from build123d import *

# Parameters (mm, degrees)
SKETCH1_W                = 22.575
SKETCH1_H                = 18
SKETCH1_R                = 2.75
BOSS_EXTRUDE1_DEPTH      = 4
BOSS_EXTRUDE1_DEPTH_BACK = 4
SKETCH3_R                = 3.375
SKETCH3_R_2              = 0.9905
CUT_EXTRUDE1_DEPTH       = 19
SKETCH4_W                = 13.55
SKETCH4_H                = 3.5
CUT_EXTRUDE2_DEPTH       = 19
CUT_EXTRUDE3_DEPTH       = 5.5
CHAMFER1_SIZE            = 2


with BuildPart() as part:
    # Sketch1 → Boss-Extrude1 (new body, two sides)
    with BuildSketch(Plane(origin=(0, 0, 0), x_dir=(1, 0, 0), z_dir=(0, 1, 0))) as boss_extrude1_sk:
        with Locations((-4.0875, 0)):
            Rectangle(SKETCH1_W, SKETCH1_H)
        Circle(SKETCH1_R, mode=Mode.SUBTRACT)
    extrude(amount=BOSS_EXTRUDE1_DEPTH)
    extrude(boss_extrude1_sk.sketch, amount=-BOSS_EXTRUDE1_DEPTH_BACK)

    # Sketch3 → Cut-Extrude1 (cut, through all)
    with BuildSketch(Plane.XY.offset(9)):
        with Locations((-11, 0)):
            Circle(SKETCH3_R)
        with Locations((-6.417424305, -2)):
            Circle(SKETCH3_R_2)
    extrude(amount=-CUT_EXTRUDE1_DEPTH, mode=Mode.SUBTRACT)

    # Sketch4 → Cut-Extrude2 (cut, through all)
    with BuildSketch(Plane.XY.offset(9)):
        with Locations((0.425, 2.25)):
            Rectangle(SKETCH4_W, SKETCH4_H)
    extrude(amount=-CUT_EXTRUDE2_DEPTH, mode=Mode.SUBTRACT)

    # Sketch5 → Cut-Extrude3 (cut, through all)
    with BuildSketch(Plane(origin=(0, 0.5, 0), x_dir=(-1, 0, 0), z_dir=(0, 1, 0))):
        Polygon((-1.2, -9), (-7.2, -3), (-7.2, -9), align=None)
        Polygon((-1.2, 9), (-7.2, 3), (-7.2, 9), align=None)
    extrude(amount=-CUT_EXTRUDE3_DEPTH, mode=Mode.SUBTRACT)

    # Chamfer1
    chamfer1_edges = [part.edges().sort_by_distance(p)[0] for p in [
        (-15.375, 4, 0),
        (-15.375, -4, 0),
        (-6.35, 4, 0),
    ]]
    chamfer(chamfer1_edges, length=CHAMFER1_SIZE)


solid = part.part
Can you work these out from the model? Positions are in its coordinate system, mm. A direction names the side the tool comes from. Round coordinates to 2 decimals unless told otherwise and drop trailing zeros. Write each loop counter-clockwise with the first axis right and the second up, starting at its lowest first coordinate (ties: lowest second). Pieces come first, ordered by that corner, then holes. Notation, with made-up numbers: (45.5, 65.5) - (91.5, 65.5) arc R17 ccw to (91.5, 71.5) - close; hole circle Ø5 at (78, -8). An arc over 180 degrees is marked (long way). Write each question's results on one line, items separated by ' | '. Start each with the question number.
1) Suppose I cut it at B-B (x = 0). List the corners of the cut face in (y, z) for me, and give its area (4 significant figures).
2) For pin 1 Ø2 at (x, z) = (-4.5, 2.5) entering from +Y; pin 2 Ø2.5 at (x, y) = (-6.42, -2) entering from +Z; pin 3 Ø0.8 at (y, z) = (1.5, -2.5) entering from +X; pin 4 Ø4.5 at (x, z) = (0, 0) entering from +Y, each with a flat end and sliding along its axis, tell me the tip position at first contact or that it passes through.
3) We'd pull the mould along X, two halves only. Please class faces 3 (the flat face through (-7.34, 2.99, 0.13)), 4 (the cylindrical face through (-7.407, -1.956, 0.126)), 5 (the flat face through (-14.361, -3.014, 0.126)): released by +X, released by -X, zero draft, split by the parting line, or undercut.
4) Suppose I cut it at C-C (y = -2.5). List the corners of the cut face in (x, z) for me (3 decimals).
5) Suppose I cut it at A-A (z = 0). Give the number of separate pieces and of enclosed holes in the cut face, and give its area (3 significant figures).
6) Please list where these lines run through material, in increasing order: line 1 (X direction, y = -2.5, z = 6) (3 decimals); line 2 (X direction, y = -1.6, z = 0) (3 decimals); line 3 (X direction, y = -2.75, z = -1.25) (3 decimals).
7) Which directions (+Z, -Z, +X, -X, +Y, -Y) give clear straight access to the entire face, cutting with the end or side of a thin tool? Please do faces 1 (the flat face through (4.2, -1.7, -6)), 2 (the flat face through (-3, 0.5, 2)).
Here are the results:
1) outline: (-4, -9) - (0.5, -9) - (0.5, -2.75) - (-4, -2.75) - close; (-4, 2.75) - (0.5, 2.75) - (0.5, 9) - (-4, 9) - close | area: 56.25 mm2
2) pin 1: stops at y = 0.5 | pin 2: stops at z = 9 | pin 3: stops at x = -6.35 | pin 4: passes through
3) face 3: released by +X | face 4: undercut | face 5: released by -X
4) outline: (-14.875, -9) - (-13.267, -9) - (-13.267, 9) - (-14.875, 9) - close; (-8.733, -9) - (-7.272, -9) - (-7.272, 9) - (-8.733, 9) - close; (-5.562, -9) - (1.2, -9) - (7.2, -3) - (7.2, 3) - (1.2, 9) - (-5.562, 9) - close; hole circle Ø5.5 at (0, 0)
5) separate pieces: 2 | enclosed holes: 2 | area: 63.6 mm2
6) line 1: x = -14.875 to -13.267, -8.733 to -7.272, -5.562 to 4.2 | line 2: x = -15.375 to -13.972, -8.028 to -7.324, -5.511 to -2.75, 2.75 to 7.2 | line 3: x = -14.625 to -12.957, -9.043 to -7.064, -5.77 to -2.449, 2.449 to 7.2
7) face 1: -Z, +X, +Y, -Y | face 2: +Z, -Z, +X, +Y
